Model file for the job. Use its own axes, mm. Face numbers are marked on the shaded views. A direction names the side the tool comes from. Give positions to 0.01 mm unless a question says otherwise; leave off trailing zeros. Order: outer loops, then holes, each group sorted by start corner. A loop starts at its lowest first (then second) coordinate and runs counter-clockwise, first axis right, second up. Notation, with made-up numbers: (52.25, 75.25) - (63.25, 75.25) arc R30 cw to (63.25, 114.25) - close; hole circle Ø2 at (7, 74.25). An arc over 180 degrees is marked (long way). Return JSON: item names as keys, results as strings. Group by question number.
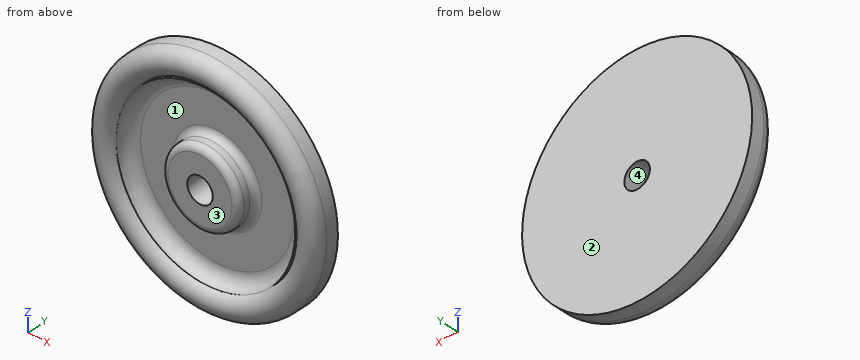
from build123d import *

# Parameters (mm, degrees)
F2_R = 3.175


with BuildPart() as f1:
    # F0 (on Right) → F1 (revolve)
    with BuildSketch(Plane.YZ):
        with BuildLine():
            Line((-12.7, 6.35), (0, 6.35))
            Line((0, 6.35), (0, 57.15))
            Line((0, 57.15), (-6.35, 57.15))
            ThreePointArc((-6.35, 57.15), (-12.7, 50.8), (-6.35, 44.45))
            Line((-6.35, 44.45), (-9.525, 44.45))
            ThreePointArc((-9.525, 44.45), (-5.034872, 42.590128), (-3.175, 38.1))
            Line((-3.175, 38.1), (-3.175, 19.05))
            Line((-3.175, 19.05), (-12.7, 19.05))
            Line((-12.7, 19.05), (-12.7, 6.35))
        make_face()
    revolve(axis=Axis((0, 10.707394, 0), (0, 1, 0)))

    # F2
    f2_edges = [f1.edges().sort_by_distance(p)[0] for p in [
        (0, -3.175, -19.05),
        (0, -12.7, -19.05),
    ]]
    fillet(f2_edges, radius=F2_R)


solid = f1.part
(1) Slice it at B-B (x = 0). Give the cut face in (y, z) (3 decimals).
(2) Drop flat-ended pins along their axis: pin 1 Ø2 at (x, z) = (-34.5, -34) entering from +Y; pin 2 Ø12 at (x, z) = (-12.5, -38.5) entering from -Y; pin 3 Ø1 at (x, z) = (43, -36) entering from -Y; pin 4 Ø4 at (x, z) = (-18, -0.5) entering from -Y. Give the stop position or say it passes through.
(3) Slice it at A-A (z = 0). Give the cut face in (x, y) (3 decimals), and give its area (3 significant figures).
(4) Pull direction X, two halves, no side cores. Call the marked faces 3 and 4: released by +X, released by -X, zero draft, split by the parting line, or undercut.
(5) 3-axis set-ups, long thin cutter, end or side, ignore diameter. For the marked faces 1 and 2: which of +Z, -Z, +X, -X, +Y, -Y reach the whole face in a straight line?
(6) Drill centre lines: L1, parallel to Z at x = -9.5, y = -8; L2, parallel to X at y = -5.75, z = 0; L3, parallel to X at y = -6.25, z = 29. Where is each one in solid material? Low to high.
Result set:
{
 "1": {"outline": "(-12.7, -15.875) arc R3.175 ccw to (-9.525, -19.05) - (-6.35, -19.05) arc R3.175 cw to (-3.175, -22.225) - (-3.175, -38.1) arc R6.35 cw to (-9.525, -44.45) - (-6.35, -44.45) arc R6.35 ccw to (-6.35, -57.15) - (0, -57.15) - (0, -6.35) - (-12.7, -6.35) - close; (-12.7, 6.35) - (0, 6.35) - (0, 57.15) - (-6.35, 57.15) arc R6.35 ccw to (-6.35, 44.45) - (-9.525, 44.45) arc R6.35 cw to (-3.175, 38.1) - (-3.175, 22.225) arc R3.175 cw to (-6.35, 19.05) - (-9.525, 19.05) arc R3.175 ccw to (-12.7, 15.875) - close"},
 "2": {"pin 1": "stops at y = 0", "pin 2": "stops at y = -11", "pin 3": "stops at y = -10.53", "pin 4": "stops at y = -12.7"},
 "3": {"outline": "(-57.15, -6.35) arc R6.35 ccw to (-44.45, -6.35) - (-44.45, -9.525) arc R6.35 cw to (-38.1, -3.175) - (-22.225, -3.175) arc R3.175 cw to (-19.05, -6.35) - (-19.05, -9.525) arc R3.175 ccw to (-15.875, -12.7) - (-6.35, -12.7) - (-6.35, 0) - (-57.15, 0) - close; (6.35, -12.7) - (15.875, -12.7) arc R3.175 ccw to (19.05, -9.525) - (19.05, -6.35) arc R3.175 cw to (22.225, -3.175) - (38.1, -3.175) arc R6.35 cw to (44.45, -9.525) - (44.45, -6.35) arc R6.35 ccw to (57.15, -6.35) - (57.15, 0) - (6.35, 0) - close", "area": "789 mm²"},
 "4": {"face 3": "zero draft", "face 4": "undercut"},
 "5": {"face 1": "-Y", "face 2": "+Z, -Z, +X, -X, +Y"},
 "6": {"L1": "z = -56.13 to -43.65, -43.42 to -43.23, -16.51 to 16.51, 43.23 to 43.42, 43.65 to 56.13", "L2": "x = -57.15 to -43.21, -19.11 to -6.35, 6.35 to 19.11, 43.21 to 57.15", "L3": "x = -49.25 to -32.48, 32.48 to 49.25"}
}
